For this review, take the finished solid that the model builds, in its own axes (mm). A direction names the side the tool comes from. Round coordinates to 2 decimals unless told otherwise and drop trailing zeros. Write each loop counter-clockwise with the first axis right and the second up, starting at its lowest first coordinate (ties: lowest second). Pieces come first, ordered by that corner, then holes. Notation, with made-up numbers: M 8,75 L 16,75 A15 ccw 16,83 Z; hole C 72.25,82.25 d3. An arc over 180 degrees is marked long. Use one line per item in the form item = value. Start each with the question number.
Item 1: Add section A-A (y = -22.5). State the section outline as (x, z) points.
Item 2: Add section D-D (x = -17). State the section outline as (y, z) points, and give its area (3 significant figures).
Item 3: Add section B-B (z = 9). State the section outline as (x, y) points.
Item 4: For faces 4 (the cylindrical face through (-36.2, -23.65, 8.03)), 5 (the flat face through (33.19, -30.95, 4.93)), 6 (the cylindrical face through (46.655, -15.229, 5.07)), list the 3-axis set-ups (+Z, -Z, +X, -X, +Y, -Y) from which the entire face can be reached by the end or side of a thin tool; tool diameter is ignored.
Item 5: For line 1 (X direction, y = -22.5, z = 1.2); line 2 (X direction, y = -31.5, z = 6.5); line 3 (Y direction, x = 36.5, z = 9.5), list the stretches that pass through material, from the lowest coordinate up. Write a range as [from, to].
Item 6: For P1, Ø6, axis at x = 17, z = 8, coming from the -Y side; P2, Ø1.9, axis at x = -38.97, y = -22.5, coming from the +Z side; P3, Ø3, axis at y = -14.5, z = 5, coming from the +X side; P4, Ø3, axis at x = 38.5, y = -21.5, coming from the +Z side, all flat-tipped, find the tip position at first contact; note any pin that passes through.
Item 7: Draft analysis for pull direction Y (two halves, no side actions). For faces 1 (the flat face through (3, -37, 0)), 2 (the cylindrical face through (-46.685, -15.29, 5.07)), 3 (the cylindrical face through (-37.445, -22.019, 2.958)), state which applies: released by +Y, released by -Y, zero draft, split by the parting line, or undercut.
Item 8: Add section C-C (y = -18.5). State the section outline as (x, z) points.
from build123d import *

# Parameters (mm, degrees)
SKETCH_1_R          = 1.6
EXTRUDE_1_DEPTH     = 10
SKETCH_2_R          = 2.5
CUT_EXTRUDE_1_DEPTH = 64.775363313
SKETCH_3_R          = 3
CUT_EXTRUDE_2_DEPTH = 4
FILLET_4_R          = 1
FILLET_5_R          = 3


with BuildPart() as part:
    # 草图1 → 凸台-拉伸1 (new body)
    with BuildSketch(Plane.XY):
        with BuildLine():
            Line((-34.426971215, -10.52538137), (-47.815237798, -14.618585236))
            ThreePointArc((-47.815237798, -14.618585236), (-43.301270189, -25), (-36.567685081, -34.099918003))
            Line((-36.567685081, -34.099918003), (-29.985501766, -27.961932763))
            ThreePointArc((-29.985501766, -27.961932763), (0, -41), (29.985501766, -27.961932763))
            Line((29.985501766, -27.961932763), (36.567685081, -34.099918003))
            ThreePointArc((36.567685081, -34.099918003), (43.301270189, -25), (47.815237798, -14.618585236))
            Line((47.815237798, -14.618585236), (34.426971215, -10.52538137))
            ThreePointArc((34.426971215, -10.52538137), (0, -36), (-34.426971215, -10.52538137))
        make_face()
        with Locations((-38.97114317, -22.5)):
            Circle(SKETCH_1_R, mode=Mode.SUBTRACT)
        with Locations((38.97114317, -22.5)):
            Circle(SKETCH_1_R, mode=Mode.SUBTRACT)
    extrude(amount=EXTRUDE_1_DEPTH)

    # 草图2 → 切除-拉伸1 (cut, through all)
    with BuildSketch(Plane.XY.offset(10)):
        with Locations((-38.252190239, -11.694868189)):
            Circle(SKETCH_2_R)
        with Locations((38.252190239, -11.694868189)):
            Circle(SKETCH_2_R)
    extrude(amount=-CUT_EXTRUDE_1_DEPTH, mode=Mode.SUBTRACT)

    # 草图3 → 切除-拉伸2 (cut)
    with BuildSketch(Plane.XY.offset(10)):
        with Locations((-38.97114317, -22.5)):
            Circle(SKETCH_3_R)
        with Locations((38.97114317, -22.5)):
            Circle(SKETCH_3_R)
    extrude(amount=-CUT_EXTRUDE_2_DEPTH, mode=Mode.SUBTRACT)

    # 圆角4
    # the kernel refuses this fillet: 1 mm, written as the material it takes off along each edge
    with BuildSketch(Plane(origin=(-34.426971215, -10.52538137, -2.466210045), x_dir=(-0.9563047559630324, -0.2923717047227467, 0), z_dir=(0, 0, 1))) as fillet_4_piece_1:
        with BuildLine():
            CenterArc((0.986484018, 1), FILLET_4_R, 181.548723167, 88.451276833)
            ThreePointArc((-0.013150685, 0.972972973), (-0.003287821, 0.486530921), (0, 0))
            Line((0, 0), (0.986484018, 0))
        make_face()
    extrude(amount=14.932420089, mode=Mode.SUBTRACT)
    with BuildSketch(Plane(origin=(34.426971215, -10.52538137, -2.466210045), x_dir=(-0.30526922048074906, -0.9522660883529749, 0), z_dir=(0, 0, 1))) as fillet_4_piece_2:
        with BuildLine():
            CenterArc((0.986576589, 0.999908672), FILLET_4_R, 180.774361584, 88.451276833)
            Line((-0.013332083, 0.986393924), (0, 0))
            ThreePointArc((0, 0), (0.486530921, 0.003287821), (0.973061841, 0))
        make_face()
    extrude(amount=14.932420089, mode=Mode.SUBTRACT)
    with BuildSketch(Plane(origin=(-40.642952128, -12.425797451, -2.135254916), x_dir=(0.42737008907787555, -0.9040767705021342, 0), z_dir=(0, 0, 1)), Plane(origin=(35.861428349, -10.963938927, -2.135254916), x_dir=(-0.1512474530257889, -0.9884959321885001, 0), z_dir=(0, 0, 1))) as fillet_4_piece_3:
        with BuildLine():
            CenterArc((0.866217493, -0.989523837), FILLET_4_R, 98.3007748, 73.398450401)
            Line((-0.123306344, -0.845154255), (0, 0))
            ThreePointArc((0, 0), (0.360923955, -0.026190408), (0.721847911, 0))
        make_face()
    extrude(amount=14.270509831, mode=Mode.SUBTRACT)
    with BuildSketch(Plane(origin=(-35.861428349, -10.963938927, -2.135254916), x_dir=(0.9563047559630329, 0.29237170472274493, 0), z_dir=(0, 0, 1)), Plane(origin=(40.642952128, -12.425797451, -2.135254916), x_dir=(0.9563047559630371, -0.2923717047227312, 0), z_dir=(0, 0, 1))) as fillet_4_piece_4:
        with BuildLine():
            CenterArc((0.854101966, -1), FILLET_4_R, 90, 73.398450401)
            ThreePointArc((-0.104212881, -0.714285714), (-0.026190408, -0.360923955), (0, 0))
            Line((0, 0), (0.854101966, 0))
        make_face()
    extrude(amount=14.270509831, mode=Mode.SUBTRACT)

    # 圆角5
    fillet_5_edges = [part.edges().sort_by_distance(p)[0] for p in [
        (-47.815237798, -14.618585236, 5),
        (47.815237798, -14.618585236, 5),
        (36.567685081, -34.099918003, 5),
        (29.985501766, -27.961932763, 5),
        (-29.985501766, -27.961932763, 5),
        (-36.567685081, -34.099918003, 5),
    ]]
    fillet(fillet_5_edges, radius=FILLET_5_R)


solid = part.part
Calculated:
q1.outline = M -44.65,0 L -40.57,0 L -40.57,6 L -41.97,6 L -41.97,10 L -44.65,10 Z; M -37.37,0 L -28.1,0 L -28.1,10 L -35.97,10 L -35.97,6 L -37.37,6 Z; M 28.1,0 L 37.37,0 L 37.37,6 L 35.97,6 L 35.97,10 L 28.1,10 Z; M 40.57,0 L 44.65,0 L 44.65,10 L 41.97,10 L 41.97,6 L 40.57,6 Z
q2.outline = M -37.31,0 L -31.73,0 L -31.73,10 L -37.31,10 Z
q2.area = 55.8 mm^2
q3.outline = M -46.78,-17.64 A50 ccw -38.67,-31.7 A3 ccw -34.3,-31.99 L -32.1,-29.94 A3 cw -28.01,-29.94 A41 ccw 28.01,-29.94 A3 cw 32.1,-29.94 L 34.3,-31.99 A3 ccw 38.67,-31.7 A50 ccw 46.78,-17.64 A3 ccw 44.85,-13.71 L 41.46,-12.68 A1 ccw 40.33,-13.08 A2.5 cw 35.75,-11.68 A1 ccw 35.2,-10.78 A1 ccw 34.13,-11.45 A36 cw -34.13,-11.45 A1 ccw -35.2,-10.78 A1 ccw -35.75,-11.68 A2.5 cw -40.33,-13.08 A1 ccw -41.46,-12.68 L -44.85,-13.71 A3 ccw Z; hole C -38.97,-22.5 d6; hole C 38.97,-22.5 d6
q4.face_4 = +Z
q4.face_5 = +Z, -Z, -Y
q4.face_6 = +Z, -Z, +X
q5.line_1 = [-44.65, -40.57], [-37.37, -28.1], [28.1, 37.37], [40.57, 44.65]
q5.line_2 = [-38.83, -33.78], [-26.24, -17.43], [17.43, 26.24], [33.78, 38.83]
q5.line_3 = [-32.79, -24.2], [-20.8, -13.48]
q6.P1 = -38.54
q6.P2 = through
q6.P3 = 46.92
q6.P4 = 6
q7.face_1 = zero draft
q7.face_2 = split by the parting line
q7.face_3 = undercut
q8.outline = M -46.45,0 L -30.88,0 L -30.88,10 L -46.45,10 Z; M 30.88,0 L 46.45,0 L 46.45,10 L 30.88,10 Z
